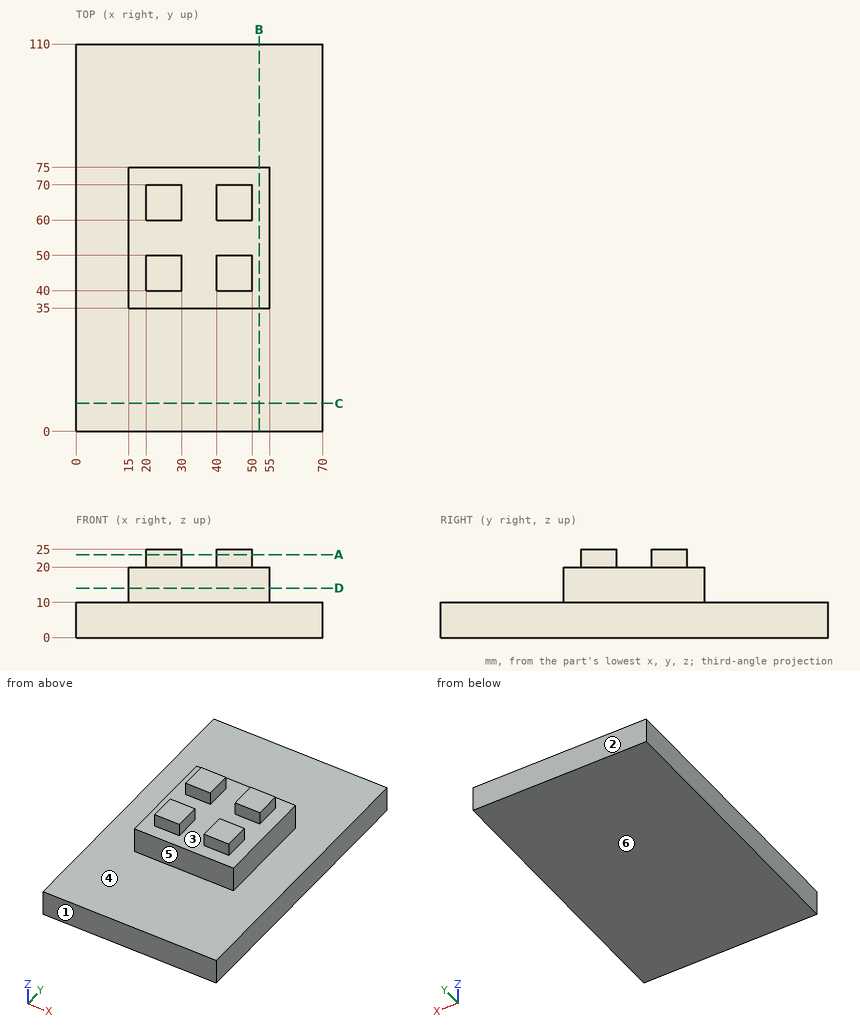
Input: dimensioned drawing with shaded views. Units: mm. Origin: part minimum x, y, z. A direction names the side the tool comes from. Coordinates: 2 decimals unless noted, no trailing zeros. Order: outer loops, then holes, each group sorted by start corner. A loop starts at its lowest first (then second) coordinate and runs counter-clockwise, first axis right, second up. Notation, with made-up numbers: (-26, 45.25) - (1, 45.25) arc R25 cw to (1, 62.25) - close; hole circle Ø8 at (-5, -6.75). An arc over 180 degrees is marked (long way). Put each result on its own line as item: value.
1. Cut plane A-A on z = 23.5. Return the cut outline in (x, y), then the cut area to 3 significant figures.
Report:
outline: (20, 40) - (30, 40) - (30, 50) - (20, 50) - close; (20, 60) - (30, 60) - (30, 70) - (20, 70) - close; (40, 40) - (50, 40) - (50, 50) - (40, 50) - close; (40, 60) - (50, 60) - (50, 70) - (40, 70) - close
area: 400 mm2
2. Reachability of the marked faces 5 and 6 from +Z, -Z, +X, -X, +Y, -Y: full face, straight path, thin tool, end or side. Return the list, or none.
Report:
face 5: +Z, +X, -X, -Y
face 6: -Z, +X, -X, +Y, -Y
3. Line query: line 1 along X through (y, z) = (44.5, 15.25); line 2 along Y through (x, z) = (18.5, 11.25); line 3 along Z through (x, y) = (51, 4). Output: solid intervals per line, ascending.
Report:
line 1: x = 15 to 55
line 2: y = 35 to 75
line 3: z = 0 to 10
4. Cut plane B-B on x = 52. Return the cut outline in (y, z).
Report:
outline: (0, 0) - (110, 0) - (110, 10) - (75, 10) - (75, 20) - (35, 20) - (35, 10) - (0, 10) - close
5. Contact query for flat-ended pins moving along their axis: pin 1 Ø8 at (x, y) = (50.5, 29) entering from +Z; pin 2 Ø5 at (x, z) = (43, 15.5) entering from +Y; pin 3 Ø2.5 at (y, z) = (47.5, 23.5) entering from -X; pin 4 Ø10 at (y, z) = (95.5, 15.5) entering from -X. Output: stop coordinate, or through.
Report:
pin 1: stops at z = 10
pin 2: stops at y = 75
pin 3: stops at x = 20
pin 4: passes through
6. Cut plane D-D on z = 14. Return the cut outline in (x, y).
Report:
outline: (15, 35) - (55, 35) - (55, 75) - (15, 75) - close
7. Cut plane C-C on y = 8. Return the cut outline in (x, z), then the cut area to 3 significant figures.
Report:
outline: (0, 0) - (70, 0) - (70, 10) - (0, 10) - close
area: 700 mm2
8. Draft query along Y for the marked faces 1, 2, 3 and 4. Return one class per face: pulls with the +Y half, pulls with the -Y half, needs draft (parallel to the pull), parting line crosses it, or undercut.
Report:
face 1: pulls with the -Y half
face 2: pulls with the +Y half
face 3: undercut
face 4: needs draft
